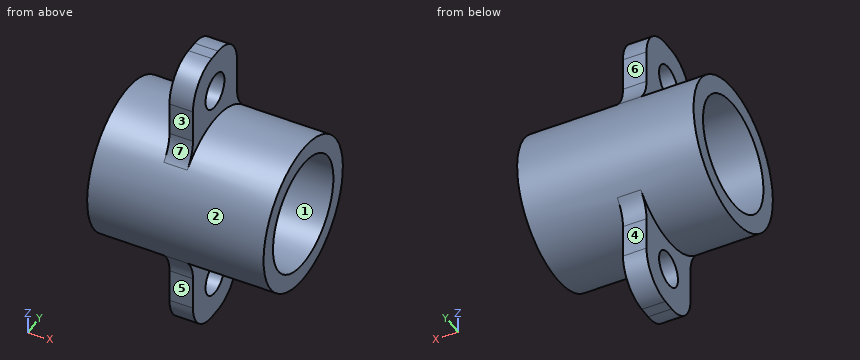
from build123d import *

# Parameters (mm, degrees)
SKETCH1_R           = 6.3
BOSS_EXTRUDE1_DEPTH = 7.5
SKETCH26_R          = 1.5
BOSS_EXTRUDE3_DEPTH = 2
FILLET1_R           = 3
SKETCH24_R          = 4.8
CUT_EXTRUDE1_DEPTH  = 16


with BuildPart() as part:
    # Sketch1 → Boss-Extrude1 (new body, symmetric)
    with BuildSketch(Plane(origin=(0, 0, 0), x_dir=(0, 0, -1), z_dir=(1, 0, 0))):
        Circle(SKETCH1_R)
    extrude(amount=BOSS_EXTRUDE1_DEPTH, both=True)

    # Sketch26 → Boss-Extrude3 (add)
    with BuildSketch(Plane(origin=(0, 0, 0), x_dir=(0, 0, -1), z_dir=(1, 0, 0))):
        with BuildLine():
            Line((5.238320341, 3.5), (12.5, 3.5))
            Line((12.5, 3.5), (12.5, -3.5))
            Line((12.5, -3.5), (5.238320341, -3.5))
            ThreePointArc((5.238320341, -3.5), (6.3, 0), (5.238320341, 3.5))
        make_face()
        with Locations((9, 0)):
            Circle(SKETCH26_R, mode=Mode.SUBTRACT)
        with BuildLine():
            Line((-5.238320341, -3.5), (-12.5, -3.5))
            Line((-12.5, -3.5), (-12.5, 3.5))
            Line((-12.5, 3.5), (-5.238320341, 3.5))
            ThreePointArc((-5.238320341, 3.5), (-6.3, 0), (-5.238320341, -3.5))
        make_face()
        with Locations((-9, 0)):
            Circle(SKETCH26_R, mode=Mode.SUBTRACT)
    extrude(amount=-BOSS_EXTRUDE3_DEPTH)

    # Fillet1
    fillet1_edges = [part.edges().sort_by_distance(p)[0] for p in [
        (-1, -3.5, 12.5),
        (-1, 3.5, 12.5),
        (-1, 3.5, 5.238320341),
        (-1, -3.5, 5.238320341),
        (-1, -3.5, -5.238320341),
        (-1, 3.5, -5.238320341),
        (-1, 3.5, -12.5),
        (-1, -3.5, -12.5),
    ]]
    fillet(fillet1_edges, radius=FILLET1_R)

    # Sketch24 → Cut-Extrude1 (cut, through all)
    with BuildSketch(Plane.ZY.offset(7.5)):
        Circle(SKETCH24_R)
    extrude(amount=-CUT_EXTRUDE1_DEPTH, mode=Mode.SUBTRACT)


solid = part.part
Part model, mm, in its own coordinate system. Face numbers are marked on the shaded views. A direction names the side the tool comes from. Give positions to 0.01 mm unless a question says otherwise; leave off trailing zeros. Loops run counter-clockwise (first coordinate to the right, second up) from the corner with the lowest first, then second, coordinate; pieces in that order, holes last. Notation, with made-up numbers: M -1,44.25 L 27,44.25 A17 ccw 27,65.25 Z; hole C 30,28.5 d4. An arc over 180 degrees is marked long. Put each result on its own line as item: value. Start each with the question number.
1) Saw through at B-B (z = 0). List the corners of the cut face in (x, y), then the cut area to 3 significant figures.
2) Pull direction Y, two halves, no side cores. Call the marked faces 1, 2 and 3: +Y half, -Y half, draft (parallel to the pull), parting line (faces both ways), or undercut.
3) 3-axis set-ups, long thin cutter, end or side, ignore diameter. For the marked faces 4, 5, 6 and 7: which of +Z, -Z, +X, -X, +Y, -Y reach the whole face in a straight line?
4) Flat gauge pins, fed straight in: pin 1 (1.5 mm diameter, centred on x = -4, y = 1, fed in from +Z); pin 2 (3 mm diameter, centred on y = 2, z = -7, fed in from -X); pin 3 (0.6 mm diameter, centred on x = -0.5, z = -8, fed in from +Y); pin 4 (1 mm diameter, centred on x = -2, y = -3.5, fed in from -Z). Where does each tip first touch, or does it go through?
5) Saw through at C-C (z = -9). List the corners of the cut face in (x, y), then the cut area to 3 significant figures.
6) Saw through at A-A (y = 0). List the corners of the cut face in (x, z).
7) Saw through at D-D (x = 6). List the corners of the cut face in (y, z).
8) Probe probe 1 along Y at (x, z) = (-1.1, -9); probe 2 along Z at (x, y) = (0.75, -0.25). List the from-to ranges inside material, lowest first.
Numbers:
1. outline: M -7.5,-6.3 L 7.5,-6.3 L 7.5,-4.8 L -7.5,-4.8 Z; M -7.5,4.8 L 7.5,4.8 L 7.5,6.3 L -7.5,6.3 Z
1. area: 45.0 mm^2
2. face 1: undercut
2. face 2: parting line
2. face 3: -Y half
3. face 4: -Z, +X, -X, +Y
3. face 5: -Z, +X, -X, -Y
3. face 6: +Z, +X, -X, +Y
3. face 7: +Z, +X, -X, -Y
4. pin 1: z = 6.3
4. pin 2: x = -7.5
4. pin 3: y = 3.5
4. pin 4: z = -11.16
5. outline: M -2,-3.5 L 0,-3.5 L 0,-1.5 L -2,-1.5 Z; M -2,1.5 L 0,1.5 L 0,3.5 L -2,3.5 Z
5. area: 8.00 mm^2
6. outline: M -7.5,-6.3 L -2,-6.3 L -2,-7.5 L 0,-7.5 L 0,-6.3 L 7.5,-6.3 L 7.5,-4.8 L -7.5,-4.8 Z; M -7.5,4.8 L 7.5,4.8 L 7.5,6.3 L 0,6.3 L 0,7.5 L -2,7.5 L -2,6.3 L -7.5,6.3 Z; M -2,-12.5 L 0,-12.5 L 0,-10.5 L -2,-10.5 Z; M -2,10.5 L 0,10.5 L 0,12.5 L -2,12.5 Z
7. outline: C 0,0 d12.6; hole C 0,0 d9.6
8. probe 1: -3.5 to -1.5, 1.5 to 3.5
8. probe 2: -6.3 to -4.79, 4.79 to 6.3
